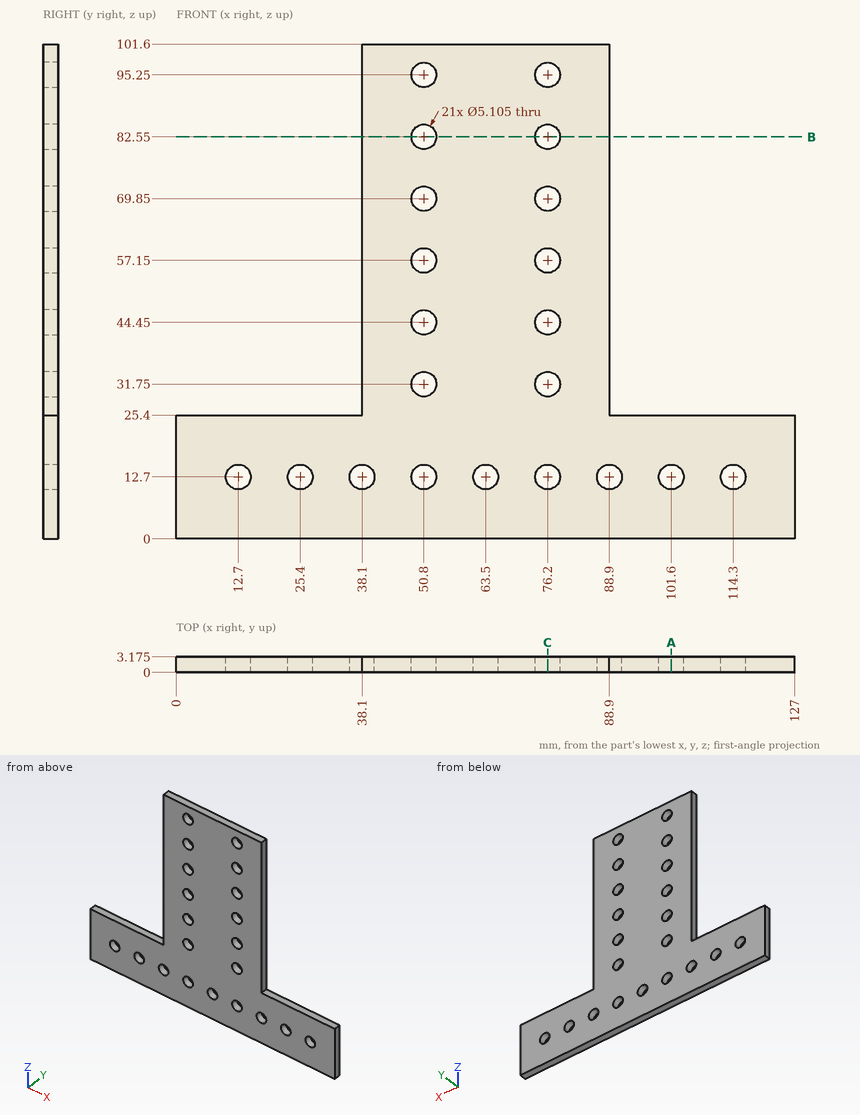
Design review of the part shown in the three views and the two pictorial views. Dimensions are in mm from the part's minimum x, y and z. Coordinates: 2 decimals unless noted, no trailing zeros. Write each loop counter-clockwise with the first axis right and the second up, starting at its lowest first coordinate (ties: lowest second). Pieces come first, ordered by that corner, then holes.
(1) Add section C-C on x = 76.2. Count the separate pieces of the cut face and the enclosed holes in it, then the cut area to 3 significant figures.
(2) Add section A-A on x = 101.6. Give the boundary of the cut face in (y, z) (1 decimal).
(3) Wall thickness on probe 1 along X at (y, z) = (1.45, 82.55); probe 2 along Z at (x, y) = (117.5, 2.1): over which ranges is each line inside the solid? List them lowest first.
(4) For pin 1 Ø1 at (y, z) = (2.5, 76.5) entering from +X; pin 2 Ø1 at (y, z) = (1.5, 78) entering from -X; pin 3 Ø1.6 at (x, y) = (104.5, 2) entering from +Z, all flat-tipped, find the tip position at first contact; note any pin that passes through.
(5) Add section B-B on z = 82.55. Give the boundary of the cut face in (x, y) (1 decimal).
Answer sheet:
1. separate pieces: 8
1. enclosed holes: 0
1. area: 209 mm2
2. outline: (0, 0) - (3.2, 0) - (3.2, 10.1) - (0, 10.1) - close; (0, 15.3) - (3.2, 15.3) - (3.2, 25.4) - (0, 25.4) - close
3. probe 1: x = 38.1 to 48.25, 53.35 to 73.65, 78.75 to 88.9
3. probe 2: z = 0 to 25.4
4. pin 1: stops at x = 88.9
4. pin 2: stops at x = 38.1
4. pin 3: stops at z = 25.4
5. outline: (38.1, 0) - (48.2, 0) - (48.2, 3.2) - (38.1, 3.2) - close; (53.4, 0) - (73.6, 0) - (73.6, 3.2) - (53.4, 3.2) - close; (78.8, 0) - (88.9, 0) - (88.9, 3.2) - (78.8, 3.2) - close
